Input: part model. Units: mm. Frame: model coordinates. A direction names the side the tool comes from. Coordinates: 2 decimals unless noted, no trailing zeros. Write each loop counter-clockwise with the first axis right and the second up, starting at its lowest first coordinate (ties: lowest second). Pieces come first, ordered by that corner, then holes. Notation, with made-up numbers: M -36.75,65.25 L 7.25,65.25 A9 ccw 7.25,72.25 Z; hole C 38,1 d9. An arc over 180 degrees is marked long. Use one line per item in the form item = value.
from build123d import *

# Parameters (mm, degrees)
BOSS_EXTRUDE1_DEPTH = 8
SKETCH2_R           = 4.95
BOSS_EXTRUDE2_DEPTH = 29
FILLET1_R           = 2
SKETCH3_R           = 1.55
CUT_EXTRUDE1_DEPTH  = 34.544199697
FILLET2_R           = 1
CUT_EXTRUDE3_START  = -2
SKETCH5_R           = 2.0875
CUT_EXTRUDE3_DEPTH  = 2


with BuildPart() as part:
    # Sketch1 → Boss-Extrude1 (new body)
    with BuildSketch(Plane(origin=(0, 0, 0), x_dir=(1, 0, 0), z_dir=(0, 1, 0))):
        Polygon((7.3, -4.214656965), (7.3, 4.214656965), (0, 8.42931393), (-7.3, 4.214656965), (-7.3, -4.214656965), (0, -8.42931393), align=None)
    extrude(amount=BOSS_EXTRUDE1_DEPTH)

    # Sketch2 → Boss-Extrude2 (add)
    with BuildSketch(Plane.XZ):
        with Locations(Location((0, 0, 0), (0, 0, 90))):
            Circle(SKETCH2_R)
        with BuildLine():
            Line((-1.5, 1.451776928), (-1.5, -1.451776928))
            ThreePointArc((-1.5, -1.451776928), (2.0875, 0), (-1.5, 1.451776928))
        make_face(mode=Mode.SUBTRACT)
    extrude(amount=BOSS_EXTRUDE2_DEPTH)

    # Fillet1
    fillet1_edges = [part.edges().sort_by_distance(p)[0] for p in [
        (0, 0, -4.95),
    ]]
    fillet(fillet1_edges, radius=FILLET1_R)

    # Sketch3 → Cut-Extrude1 (cut, through all)
    with BuildSketch(Plane(origin=(7.3, 0, 0), x_dir=(0, 0, -1), z_dir=(1, 0, 0))):
        with Locations((-0.085343035, 3.85)):
            Circle(SKETCH3_R)
    extrude(amount=-CUT_EXTRUDE1_DEPTH, mode=Mode.SUBTRACT)

    # Fillet2
    fillet2_edges = [part.edges().sort_by_distance(p)[0] for p in [
        (0, 4, 8.42931393),
        (-7.3, 4, 4.214656965),
        (-7.3, 4, -4.214656965),
        (0, 4, -8.42931393),
        (7.3, 4, -4.214656965),
        (7.3, 4, 4.214656965),
        (3.65, 8, -6.321985448),
        (-3.65, 8, -6.321985448),
        (-7.3, 8, 0),
        (-3.65, 8, 6.321985448),
        (3.65, 8, 6.321985448),
        (7.3, 8, 0),
    ]]
    fillet(fillet2_edges, radius=FILLET2_R)

    # Sketch5 → Cut-Extrude3 (cut)
    with BuildSketch(Plane.XZ.offset(29).offset(CUT_EXTRUDE3_START)):
        with Locations(Location((0, 0, 0), (0, 0, 135.935955789))):
            Circle(SKETCH5_R)
    extrude(amount=CUT_EXTRUDE3_DEPTH, mode=Mode.SUBTRACT)


solid = part.part
(1) Section query A-A on y = 3.85. Return the cut outline in (x, z), plus the area to 3 significant figures.
Computed:
outline = M -7.3,-3.64 A1 ccw -6.8,-4.5 L -0.5,-8.14 A1 ccw 0.5,-8.14 L 6.8,-4.5 A1 ccw 7.3,-3.64 L 7.3,-1.46 L -7.3,-1.46 Z; M -7.3,1.64 L 7.3,1.64 L 7.3,3.64 A1 ccw 6.8,4.5 L 0.5,8.14 A1 ccw -0.5,8.14 L -6.8,4.5 A1 ccw -7.3,3.64 Z
area = 139 mm^2
(2) Section query B-B on z = 0. Return the cut outline in (x, y).
Computed:
outline = M -7.3,0 L -6.95,0 A2 cw -4.95,-2 L -4.95,-29 L -2.09,-29 L -2.09,-27 L -1.5,-27 L -1.5,0 L 2.09,0 L 2.09,-29 L 4.95,-29 L 4.95,-2 A2 cw 6.95,0 L 7.3,0 L 7.3,2.3 L -7.3,2.3 Z; M -7.3,5.4 L 7.3,5.4 L 7.3,7 A1 ccw 6.3,8 L -6.3,8 A1 ccw -7.3,7 Z
(3) Pull-direction query (Y, two-part tool) for faces 3 (the cylindrical face through (3.55, 7.7, 6.05)), 4 (the flat face through (-7.3, 2, 0)), 5 (the cylindrical face through (0.102, 2.337, 0.421)); classes: pulls with the +Y half, pulls with the -Y half, needs draft (parallel to the pull), parting line crosses it, or undercut.
Computed:
face_3 = pulls with the +Y half
face_4 = needs draft
face_5 = undercut
(4) Section query D-D on y = -1. Return the cut outline in (x, z) (1 decimal), plus the area to 3 significant figures.
Computed:
outline = C 0,0 d10.4; hole M -1.5,-1.5 A2.1 ccw long -1.5,1.5 Z
area = 73.0 mm^2
(5) Set-up query: faces 1 (the cylindrical face through (-1.49, -15.31, 4.72)), 2 (the cylindrical face through (-7.162, 3.549, -4.144)). Return all of +Z, -Z, +X, -X, +Y, -Y with unobstructed straight access to the full face (end or side cutting, diameter ignored); none if empty.
Computed:
face_1 = -Y
face_2 = -Z, -X, +Y, -Y
(6) Line query: probe 1 along X at (y, z) = (-9.75, 0); probe 2 along Y at (x, z) = (3.75, 0); probe 3 along Y at (x, z) = (-3.5, -0.5). Output: solid intervals per line, ascending.
Computed:
probe_1 = -4.95 to -1.5, 2.09 to 4.95
probe_2 = -29 to 2.3, 5.4 to 8
probe_3 = -29 to 2.41, 5.29 to 8
(7) First-contact query: pin 1 Ø2 at (y, z) = (-19.5, -4.5) entering from +X; pin 2 Ø1 at (x, y) = (-0.5, -23.5) entering from -Z; pin 3 Ø5 at (x, y) = (1, -21) entering from +Z; pin 4 Ø5 at (y, z) = (3.85, 0.09) entering from +X. Flat tips, straight axial feed; report the tip coordinate or a pass-through.
Computed:
pin_1 = 3.5
pin_2 = -4.95
pin_3 = 4.95
pin_4 = 7.3
